Check sheet for the modelled part. Datum: model origin and axes. Units: mm. Round coordinates to 2 decimals unless told otherwise and drop trailing zeros. Loops run counter-clockwise (first coordinate to the right, second up) from the corner with the lowest first, then second, coordinate; pieces in that order, holes last. Notation, with made-up numbers: (72.25, -21.5) - (99.25, -21.5) arc R5 cw to (99.25, -17.5) - close; hole circle Ø5 at (0, 61.5). An arc over 180 degrees is marked (long way). Put each result on its own line as item: value. Start each with the question number.
```python
from build123d import *

# Parameters (mm, degrees)
SKETCH_1_R      = 2
EXTRUDE_1_DEPTH = 3
FILLET_1_R      = 2


with BuildPart() as part:
    # 草图1 → 凸台-拉伸1 (new body)
    with BuildSketch(Plane(origin=(0, 0, 0), x_dir=(1, 0, 0), z_dir=(0, 1, 0))):
        Polygon((0, 0), (0, -50), (140, -50), (140, 50), (0, 50), align=None)
        with Locations(Location((16.4, -30.1, 0), (0, 0, 270))):
            Circle(SKETCH_1_R, mode=Mode.SUBTRACT)
        with Locations(Location((16.4, 19.9, 0), (0, 0, 270))):
            Circle(SKETCH_1_R, mode=Mode.SUBTRACT)
        with Locations(Location((126.4, 28.5, 0), (0, 0, 270))):
            Circle(SKETCH_1_R, mode=Mode.SUBTRACT)
        with Locations(Location((126.4, -30.1, 0), (0, 0, 270))):
            Circle(SKETCH_1_R, mode=Mode.SUBTRACT)
    extrude(amount=EXTRUDE_1_DEPTH)

    # 圆角1
    fillet_1_edges = [part.edges().sort_by_distance(p)[0] for p in [
        (0, 1.5, 50),
        (0, 1.5, -50),
        (140, 1.5, -50),
        (140, 1.5, 50),
    ]]
    fillet(fillet_1_edges, radius=FILLET_1_R)


solid = part.part
```
Q1. Cross-section at C-C on z = -28.5. Enter the section's corners in (x, y), and give its area (3 significant figures).
Q2. Depth check by flat-ended pin: pin 1 Ø3 at (x, z) = (120.5, -12) entering from -Y. Enter the tip coordinate at first touch or a pass-through.
Q3. Cross-section at B-B on z = 30.1. Enter the section's corners in (x, y).
Q4. Cross-section at A-A on x = 126.4. Enter the section's corners in (y, z).
Q5. Draft check along Z on faces 1 (the face through (17.001, 1.479, -17.992)), 2 (the face through (128.383, 1.479, 29.84)), 3 (the face through (71, 1, -50)), 4 (the face through (69, 0, -1)). Enter one of: +Z half, -Z half, draft (parallel to the pull), parting line (faces both ways), or undercut.
Q6. Material ranges on line 1 (X direction, y = 0.95, z = 30.1); line 2 (X direction, y = 2.1, z = -28.5); line 3 (X direction, y = 2.15, z = -19.9), recorded low to high. Write a range as from..to.
Answer list:
1. outline: (0, 0) - (124.4, 0) - (124.4, 3) - (0, 3) - close; (128.4, 0) - (140, 0) - (140, 3) - (128.4, 3) - close
1. area: 408 mm2
2. pin 1: stops at y = 0
3. outline: (0, 0) - (14.4, 0) - (14.4, 3) - (0, 3) - close; (18.4, 0) - (124.4, 0) - (124.4, 3) - (18.4, 3) - close; (128.4, 0) - (140, 0) - (140, 3) - (128.4, 3) - close
4. outline: (0, -50) - (3, -50) - (3, -30.5) - (0, -30.5) - close; (0, -26.5) - (3, -26.5) - (3, 28.1) - (0, 28.1) - close; (0, 32.1) - (3, 32.1) - (3, 50) - (0, 50) - close
5. face 1: undercut
5. face 2: undercut
5. face 3: -Z half
5. face 4: draft
6. line 1: x = 0..14.4, 18.4..124.4, 128.4..140
6. line 2: x = 0..124.4, 128.4..140
6. line 3: x = 0..14.4, 18.4..140
